Could you check a few things on this model? Use its own coordinates, in mm. Face numbers are marked on the shaded views. A direction names the side the tool comes from. Coordinates: 2 decimals unless noted, no trailing zeros. Write each loop counter-clockwise with the first axis right and the second up, starting at its lowest first coordinate (ties: lowest second). Pieces come first, ordered by that corner, then holes. Notation, with made-up numbers: (84, 59.25) - (102, 59.25) arc R17 cw to (102, 79.25) - close; hole circle Ø4 at (-11.5, -0.5). An arc over 180 degrees is marked (long way). Answer as a JSON object with one key per item and string values. Group by question number.
1) On a 3-axis mill with a long thin cutter (end or side, diameter ignored), from which of +Z, -Z, +X, -X, +Y, -Y can I reach the whole of each face in a straight line? I mean the marked faces 1, 2 and 3. Say none if no direction works.
2) Will these pins go through, and if not, where does the flat tip stop? pin 1 Ø4 at (y, z) = (-8, 3.5) entering from -X; pin 2 Ø11 at (y, z) = (-6.5, 14.5) entering from +X; pin 3 Ø3 at (x, y) = (-29.21, -13.3) entering from -Z.
3) We'd pull the mould along X, two halves only. Please class the marked faces 4, 5, 6 and 7: released by +X, released by -X, zero draft, split by the parting line, or undercut.
4) If we section it at C-C (z = 12.5): Write out the boundary of the cut face in (x, y), plus the area to 3 significant figures.
5) If we section it at B-B (y = -9.5): Write out the boundary of the cut face in (x, z), plus the area to 3 significant figures.
6) Please list where these lines run through material, in increasing order: line 1 along X through (y, z) = (-13.3, 23.25); line 2 along Y through (x, z) = (-29.21, 23.25); line 3 along Y through (x, z) = (2.5, 21).
7) If we section it at A-A (x = -29.21): Write out the boundary of the cut face in (y, z).
8) If we section it at D-D (y = -16.75): Write out the boundary of the cut face in (x, z).
Autodesk Fusion 360 part; units mm, degrees
sketch "Sketch1" plane through (0, 0, 0) normal (0, 0, 1) x (1, 0, 0)
  line L0 (-25, -19.2) -> (-25, 2.3)
  line L1 (-25, 2.3) -> (17.94, 2.3)
  line L2 (17.94, 2.3) -> (17.94, -19.2)
  line L3 (17.94, -19.2) -> (-25, -19.2)
  dimension "d1" = 21.5
  dimension "d2" = 42.94
extrude "Extrude1" add sketch "Sketch1" along normal blind 28.65
shell "Shell1" thickness 0.5 removed faces 1 at (3.6267, -12.0333, 28.65)
sketch "Sketch2" plane through (17.94, 0, 0) normal (1, 0, 0) x (0, 1, 0)
  line L0 (-19.2, 0) -> (2.3, 0)
  line L1 (2.3, 0) -> (2.3, 28.65)
  line L2 (2.3, 28.65) -> (-19.2, 28.65)
  line L3 (-19.2, 28.65) -> (-19.2, 0)
  line L4 (-12.5, 8.4) -> (-4.4, 8.4)
  line L5 (-4.4, 8.4) -> (-4.4, 3.4)
  line L6 (-4.4, 3.4) -> (-12.5, 3.4)
  line L7 (-12.5, 3.4) -> (-12.5, 8.4)
  dimension "d6" = 3.4
  dimension "d7" = 8.1
  dimension "d8" = 6.7
  dimension "d9" = 6.7
  dimension "d39" = 5
extrude "Extrude2" cut sketch "Sketch2" along normal mid plane 6 contours L4 L5 L6 L7
sketch "Sketch3" plane through (17.94, 0, 0) normal (1, 0, 0) x (0, 1, 0)
  line L0 (-4.4, 8.4) -> (-4.4, 3.4)
  line L1 (-4.4, 3.4) -> (-12.5, 3.4)
  line L2 (-12.5, 3.4) -> (-12.5, 8.4)
  line L3 (-12.5, 8.4) -> (-4.4, 8.4)
  line L4 (-19.2, 0) -> (2.3, 0)
  line L5 (2.3, 0) -> (2.3, 28.65)
  line L6 (2.3, 28.65) -> (-19.2, 28.65)
  line L7 (-19.2, 28.65) -> (-19.2, 0)
  line L8 (-17.8, 28.65) -> (0.9, 28.65)
  line L9 (0.9, 28.65) -> (0.9, 20.15)
  line L10 (0.9, 20.15) -> (-17.8, 20.15)
  line L11 (-17.8, 20.15) -> (-17.8, 28.65)
  dimension "d19" = 18.7
  dimension "d20" = 1.4
  dimension "d23" = 8.5
extrude "Extrude3" add sketch "Sketch3" along normal blind 7.1 contours L6 L8 L9 L10 L11
sketch "Sketch4" plane through (0, 0, 28.65) normal (0, 0, 1) x (-1, 0, 0)
  line L0 (-17.44, 18.7) -> (24.5, 18.7)
  line L1 (24.5, 18.7) -> (24.5, -1.8)
  line L2 (24.5, -1.8) -> (-17.44, -1.8)
  line L3 (-17.44, -1.8) -> (-17.44, 18.7)
  line L4 (-17.94, 19.2) -> (-17.94, 17.8)
  line L5 (-17.94, 17.8) -> (-25.04, 17.8)
  line L6 (-25.04, 17.8) -> (-25.04, -0.9)
  line L7 (-25.04, -0.9) -> (-17.94, -0.9)
  line L8 (-17.94, -0.9) -> (-17.94, -2.3)
  line L9 (-17.94, -2.3) -> (25, -2.3)
  line L10 (25, -2.3) -> (25, 19.2)
  line L11 (25, 19.2) -> (-17.94, 19.2)
  circle A0 centre (-22.15, 3.6) radius 2.25
  circle A1 centre (-22.15, 13.3) radius 2.25
  dimension "d40" = 4.5
  dimension "d41" = 4.5
  dimension "d44" = 9.7
  dimension "d45" = 4.71
  dimension "d46" = 4.71
  dimension "d47" = 4.5
sketch "Sketch6" plane through (-25, 0, 0) normal (-1, 0, 0) x (0, -1, 0)
  line L0 (-2.3, 0) -> (19.2, 0)
  line L1 (19.2, 0) -> (19.2, 28.65)
  line L2 (19.2, 28.65) -> (-2.3, 28.65)
  line L3 (-2.3, 28.65) -> (-2.3, 0)
  line L4 (-0.9, 28.65) -> (17.8, 28.65)
  line L5 (17.8, 28.65) -> (17.8, 20.15)
  line L6 (17.8, 20.15) -> (-0.9, 20.15)
  line L7 (-0.9, 20.15) -> (-0.9, 28.65)
  dimension "d27" = 1.4
  dimension "d28" = 18.7
  dimension "d29" = 8.5
extrude "Extrude5" add sketch "Sketch6" along normal blind 7.1 contours L2 L4 L5 L6 L7
sketch "Sketch7" plane through (0, 0, 28.65) normal (0, 0, 1) x (-1, 0, 0)
  line L0 (-17.44, 18.7) -> (24.5, 18.7)
  line L1 (24.5, 18.7) -> (24.5, -1.8)
  line L2 (24.5, -1.8) -> (-17.44, -1.8)
  line L3 (-17.44, -1.8) -> (-17.44, 18.7)
  line L4 (-17.94, 19.2) -> (-17.94, 17.8)
  line L5 (-17.94, 17.8) -> (-25.04, 17.8)
  line L6 (-25.04, 17.8) -> (-25.04, -0.9)
  line L7 (-25.04, -0.9) -> (-17.94, -0.9)
  line L8 (-17.94, -0.9) -> (-17.94, -2.3)
  line L9 (-17.94, -2.3) -> (25, -2.3)
  line L10 (25, -2.3) -> (25, -0.9)
  line L11 (25, -0.9) -> (32.1, -0.9)
  line L12 (32.1, -0.9) -> (32.1, 17.8)
  line L13 (32.1, 17.8) -> (25, 17.8)
  line L14 (25, 17.8) -> (25, 19.2)
  line L15 (25, 19.2) -> (-17.94, 19.2)
  circle A0 centre (26.6, 4.1) radius 1.025
  dimension "d34" = 2.05
  dimension "d35" = 2.1
  dimension "d36" = 5
sketch "Sketch8" plane through (0, 0, 28.65) normal (0, 0, 1) x (-1, 0, 0)
  line L0 (-17.44, 18.7) -> (24.5, 18.7)
  line L1 (24.5, 18.7) -> (24.5, -1.8)
  line L2 (24.5, -1.8) -> (-17.44, -1.8)
  line L3 (-17.44, -1.8) -> (-17.44, 18.7)
  line L4 (-17.94, 19.2) -> (-17.94, 17.8)
  line L5 (-17.94, 17.8) -> (-25.04, 17.8)
  line L6 (-25.04, 17.8) -> (-25.04, -0.9)
  line L7 (-25.04, -0.9) -> (-17.94, -0.9)
  line L8 (-17.94, -0.9) -> (-17.94, -2.3)
  line L9 (-17.94, -2.3) -> (25, -2.3)
  line L10 (25, -2.3) -> (25, -0.9)
  line L11 (25, -0.9) -> (32.1, -0.9)
  line L12 (32.1, -0.9) -> (32.1, 17.8)
  line L13 (32.1, 17.8) -> (25, 17.8)
  line L14 (25, 17.8) -> (25, 19.2)
  line L15 (25, 19.2) -> (-17.94, 19.2)
  circle A0 centre (-22.15, 3.6) radius 1
  circle A1 centre (-22.15, 13.3) radius 1
  circle A2 centre (29.21, 3.6) radius 1
  circle A3 centre (29.21, 13.3) radius 1
  dimension "d48" = 2
  dimension "d49" = 2
  dimension "d50" = 4.71
  dimension "d51" = 9.7
  dimension "d52" = 4.5
  dimension "d53" = 4.71
  dimension "d54" = 2
  dimension "d55" = 2
  dimension "d56" = 9.7
  dimension "d57" = 4.71
  dimension "d58" = 4.5
  dimension "d59" = 4.71
extrude "Extrude7" cut sketch "Sketch8" against normal blind 8.65 contours A0 | A1 | A2 | A3
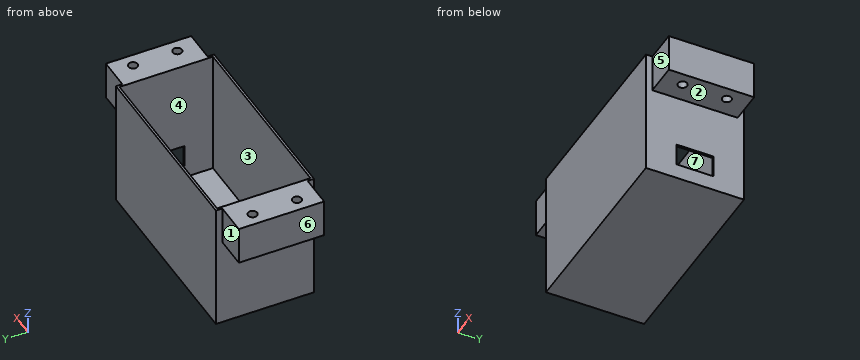
Here are the results:
{
 "1": {"face 1": "+Z, -Z, -X, +Y", "face 2": "-Z, +X, +Y, -Y", "face 3": "+Z"},
 "2": {"pin 1": "stops at x = -25", "pin 2": "stops at x = 17.94", "pin 3": "stops at z = 20.15"},
 "3": {"face 4": "undercut", "face 5": "zero draft", "face 6": "released by -X", "face 7": "undercut"},
 "4": {"outline": "(-25, -19.2) - (17.94, -19.2) - (17.94, 2.3) - (-25, 2.3) - close; hole (-24.5, -18.7) - (17.44, -18.7) - (17.44, 1.8) - (-24.5, 1.8) - close", "area": "63.4 mm²"},
 "5": {"outline": "(-32.1, 20.15) - (-25, 20.15) - (-25, 0) - (17.94, 0) - (17.94, 3.4) - (17.44, 3.4) - (17.44, 0.5) - (-24.5, 0.5) - (-24.5, 28.65) - (-32.1, 28.65) - close; (17.44, 8.4) - (17.94, 8.4) - (17.94, 20.15) - (25.04, 20.15) - (25.04, 28.65) - (17.44, 28.65) - close", "area": "168 mm²"},
 "6": {"line 1": "x = -32.1 to -30.21, -28.21 to -24.5, 17.44 to 21.15, 23.15 to 25.04", "line 2": "y = -17.8 to -14.3, -12.3 to -4.6, -2.6 to 0.9", "line 3": "y = -19.2 to -18.7, 1.8 to 2.3"},
 "7": {"outline": "(-17.8, 20.15) - (-14.3, 20.15) - (-14.3, 28.65) - (-17.8, 28.65) - close; (-12.3, 20.15) - (-4.6, 20.15) - (-4.6, 28.65) - (-12.3, 28.65) - close; (-2.6, 20.15) - (0.9, 20.15) - (0.9, 28.65) - (-2.6, 28.65) - close"},
 "8": {"outline": "(-32.1, 20.15) - (-25, 20.15) - (-25, 0) - (17.94, 0) - (17.94, 20.15) - (25.04, 20.15) - (25.04, 28.65) - (17.44, 28.65) - (17.44, 0.5) - (-24.5, 0.5) - (-24.5, 28.65) - (-32.1, 28.65) - close"}
}
